Verification items for the finished model (mm, model axes). Round coordinates to 2 decimals unless told otherwise and drop trailing zeros. Loops run counter-clockwise (first coordinate to the right, second up) from the corner with the lowest first, then second, coordinate; pieces in that order, holes last. Notation, with made-up numbers: (-20, -34) -> (39, -34) arc R34 cw to (39, 4) -> close; hole circle Ø4 at (-9, -15.75). An arc over 180 degrees is marked (long way). Write item = value, one per line. Start each with the question number.
Autodesk Inventor part; units mm, degrees
ref_plane "XZ Plane" through (0, 0, 0) normal (0, 1, 0) x (-1, 0, 0)
sketch "Sketch2" plane through (0, 0, 0) normal (0, 1, 0) x (-1, 0, 0)
  line L0 (76.2, 76.2) -> (-76.2, 76.2)
  line L1 (-76.2, 76.2) -> (-76.2, -76.2)
  line L2 (-76.2, -76.2) -> (76.2, -76.2)
  line L3 (76.2, -76.2) -> (76.2, 76.2)
  line L4 (76.2, 76.2) -> (-76.2, -76.2) construction
  line L5 (-76.2, 76.2) -> (76.2, -76.2) construction
  point P0 (0, 0)
  dimension "d0" = 152.4
extrude "Extrusion1" add sketch "Sketch2" along normal blind 12.7
sketch "Sketch3" plane through (0, 12.7, 0) normal (0, 1, 0) x (1, 0, 0)
  circle A0 centre (0, 0) radius 6.985
  dimension "d3" = 13.97
extrude "Extrusion2" cut sketch "Sketch3" against normal through all
properties part number "tableForBall"
(1) Scan lines: line 1 (Z direction, x = 0, y = 2.5) (3 decimals); line 2 (X direction, y = 4, z = -6). Record each from-to range of solid material in increasing order. Write a range as [from, to].
(2) Draft check along X on faces 1 (the cylindrical face through (-0.909, 6.439, -6.926)), 2 (the flat face through (76.2, 6, 1)), 3 (the flat face through (1, 6, -76.2)), 4 (the flat face through (-76.2, 6, -1)). Enter one of: +X half, -X half, draft (parallel to the pull), parting line (faces both ways), or undercut.
(3) Section check B-B on z = 0. Enter the section's corners in (x, y) (3 decimals), then the cut area to 3 significant figures.
(4) Section check A-A on x = 0. Enter the section's corners in (y, z) (3 decimals), then the cut area to 3 significant figures.
Computed values:
q1.line_1 = [-76.2, -6.985], [6.985, 76.2]
q1.line_2 = [-76.2, -3.58], [3.58, 76.2]
q2.face_1 = undercut
q2.face_2 = +X half
q2.face_3 = draft
q2.face_4 = -X half
q3.outline = (-76.2, 0) -> (-6.985, 0) -> (-6.985, 12.7) -> (-76.2, 12.7) -> close; (6.985, 0) -> (76.2, 0) -> (76.2, 12.7) -> (6.985, 12.7) -> close
q3.area = 1,760 mm²
q4.outline = (0, -76.2) -> (12.7, -76.2) -> (12.7, -6.985) -> (0, -6.985) -> close; (0, 6.985) -> (12.7, 6.985) -> (12.7, 76.2) -> (0, 76.2) -> close
q4.area = 1,760 mm²
